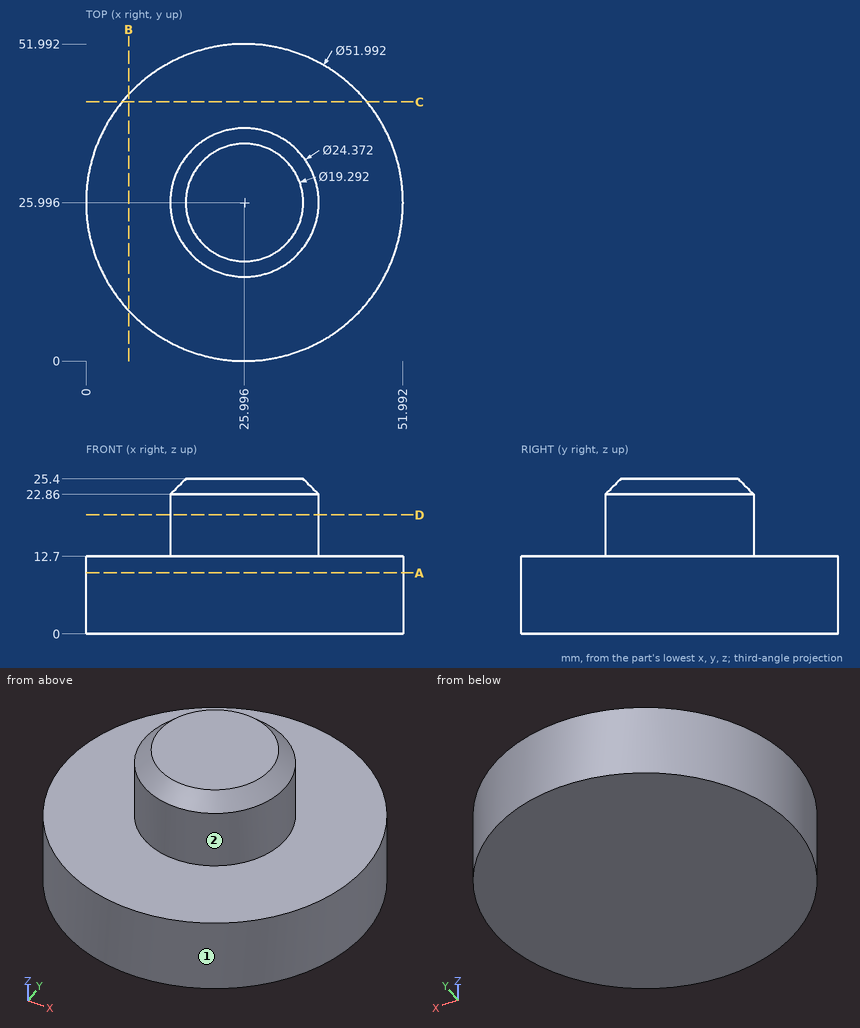
Source: three-view drawing plus pictorial views. Frame: mm from the lowest corner of the part. A direction names the side the tool comes from. Coordinates: 2 decimals unless noted, no trailing zeros. Write each loop counter-clockwise with the first axis right and the second up, starting at its lowest first coordinate (ties: lowest second). Pieces come first, ordered by that corner, then holes. Notation, with made-up numbers: (-7.75, -38) - (-2.75, -38) arc R15 cw to (-2.75, -28) - close; hole circle Ø9 at (-24, 25.5). An arc over 180 degrees is marked (long way). Return JSON: item names as keys, results as strings.
Item 1: Section query B-B (x = 7). Output: boundary loops of the cut face in (y, z).
Completed:
{"outline": "(8.25, 0) - (43.74, 0) - (43.74, 12.7) - (8.25, 12.7) - close"}
Item 2: Line query: L1, parallel to Z at x = 13, y = 43.5; L2, parallel to X at y = 25.5, z = 18.75; L3, parallel to X at y = 8.5, z = 6. Output: solid intervals per line, ascending.
Completed:
{"L1": "z = 0 to 12.7", "L2": "x = 13.82 to 38.17", "L3": "x = 6.77 to 45.22"}
Item 3: Pin query (flat end, axial travel): pin 1 Ø3 at (y, z) = (15.5, 15) entering from +X; pin 2 Ø1.5 at (y, z) = (38.5, 5) entering from -X; pin 3 Ø1 at (x, z) = (41, 6) entering from -Y. Return the tip coordinate at first contact, or that it passes through.
Completed:
{"pin 1": "stops at x = 34.22", "pin 2": "stops at x = 2.81", "pin 3": "stops at y = 4.42"}
Item 4: Section query C-C (y = 42.5). Output: boundary loops of the cut face in (x, z), and give its area (3 significant figures).
Completed:
{"outline": "(5.91, 0) - (46.08, 0) - (46.08, 12.7) - (5.91, 12.7) - close", "area": "510 mm2"}
Item 5: Reachability of the marked faces 1 and 2 from +Z, -Z, +X, -X, +Y, -Y: full face, straight path, thin tool, end or side. Return the list, or none.
Completed:
{"face 1": "+Z, -Z", "face 2": "+Z"}
Item 6: Section query D-D (z = 19.5). Output: boundary loops of the cut face in (x, y).
Completed:
{"outline": "circle Ø24.37 at (26, 26)"}
Item 7: Section query A-A (z = 10). Output: boundary loops of the cut face in (x, y).
Completed:
{"outline": "circle Ø51.99 at (26, 26)"}
